```python
from build123d import *

# Parameters (mm, degrees)
ESQUISSE1_W             = 35
ESQUISSE1_H             = 35
BOSS_EXTRU_1_DEPTH      = 800
ESQUISSE2_W             = 40
ESQUISSE2_H             = 40
ESQUISSE2_W_2           = 35
ESQUISSE2_H_2           = 35
BOSS_EXTRU_2_DEPTH      = 10
ESQUISSE7_R             = 12.5
ENL_V_MAT_EXTRU_1_DEPTH = 25


with BuildPart() as part:
    # Esquisse1 → Boss.-Extru.1 (new body)
    with BuildSketch(Plane(origin=(0, 0, 0), x_dir=(0, 0, -1), z_dir=(1, 0, 0))):
        Rectangle(ESQUISSE1_W, ESQUISSE1_H)
    extrude(amount=BOSS_EXTRU_1_DEPTH)

    # Esquisse2 → Boss.-Extru.2 (add)
    # profile 1 of 2: a face of its own
    with BuildSketch(Plane.ZY):
        Rectangle(ESQUISSE2_W, ESQUISSE2_H)
        Rectangle(ESQUISSE2_W_2, ESQUISSE2_H_2, mode=Mode.SUBTRACT)
    # profile 2 of 2: a face of its own
    with BuildSketch(Plane.ZY):
        Rectangle(ESQUISSE2_W_2, ESQUISSE2_H_2)
    extrude(amount=BOSS_EXTRU_2_DEPTH)

    # Esquisse7 → Enlèv. mat.-Extru.1 (cut)
    with BuildSketch(Plane.XY.offset(17.5)):
        with Locations((770, 0)):
            Circle(ESQUISSE7_R)
    extrude(amount=-ENL_V_MAT_EXTRU_1_DEPTH, mode=Mode.SUBTRACT)


solid = part.part
```
Work out the finished part from the listing and answer in its coordinate system (mm). A direction names the side the tool comes from. Round coordinates to 2 decimals unless told otherwise and drop trailing zeros. Write each loop counter-clockwise with the first axis right and the second up, starting at its lowest first coordinate (ties: lowest second). Pieces come first, ordered by that corner, then holes. Notation, with made-up numbers: (10, 24) - (25, 24) arc R14 cw to (25, 51) - close; hole circle Ø4 at (-12.75, 65). An arc over 180 degrees is marked (long way). Return JSON: item names as keys, results as strings. Group by question number.
Q1. Find the intervals of material crossed by L1, parallel to Y at x = 770, z = 10; L2, parallel to Z at x = 595.5, y = -8, in increasing order.
Q2. The mould has two halves that part along X. Classify faces 5 (the flat face through (-10, 0, 0)), 6 (the flat face through (770, 0, -7.5)), 7 (the flat face through (394, -17.5, 0)), 8 (the flat face through (800, 0, 0)): released by +X, released by -X, zero draft, split by the parting line, or undercut.
Q3. The part is cut by section B-B on x = 770. Write down the section's boundary in (y, z), then the cut area to 3 significant figures.
Q4. The part is cut by section D-D on x = 255.5. Write down the section's boundary in (y, z).
Q5. The part is cut by section C-C on y = 0. Write down the section's boundary in (x, z).
Q6. Each of these flat-tipped pins is pushed along its axis until it touches: pin 1 Ø2 at (x, z) = (120, -12) entering from -Y; pin 2 Ø10.5 at (x, y) = (480, 7.5) entering from -Z; pin 3 Ø17.5 at (x, z) = (560.5, -4.5) entering from +Y. Where does it stop, or does it pass through?
Q7. For faces 1 (the flat face through (394, 0, -17.5)), 2 (the flat face through (394, 0, 17.5)), 3 (the flat face through (394, 17.5, 0)), 4 (the cylindrical face through (757.512, 0.55, 5.175)), determine the directions among +Z, -Z, +X, -X, +Y, -Y from which every point of the face is accessible in a straight line to the end or side of a thin tool.
Q8. The part is cut by section A-A on z = 8. Write down the section's boundary in (x, y), then the cut area to 3 significant figures.
Solved:
{
 "1": {"L1": "-17.5 to -12.5, 12.5 to 17.5", "L2": "-17.5 to 17.5"},
 "2": {"face 5": "released by -X", "face 6": "undercut", "face 7": "zero draft", "face 8": "released by +X"},
 "3": {"outline": "(-17.5, -17.5) - (17.5, -17.5) - (17.5, 17.5) - (12.5, 17.5) - (12.5, -7.5) - (-12.5, -7.5) - (-12.5, 17.5) - (-17.5, 17.5) - close", "area": "600 mm²"},
 "4": {"outline": "(-17.5, -17.5) - (17.5, -17.5) - (17.5, 17.5) - (-17.5, 17.5) - close"},
 "5": {"outline": "(-10, -20) - (0, -20) - (0, -17.5) - (800, -17.5) - (800, 17.5) - (782.5, 17.5) - (782.5, -7.5) - (757.5, -7.5) - (757.5, 17.5) - (0, 17.5) - (0, 20) - (-10, 20) - close"},
 "6": {"pin 1": "y = -17.5", "pin 2": "z = -17.5", "pin 3": "y = 17.5"},
 "7": {"face 1": "-Z, +X, +Y, -Y", "face 2": "+Z, +X, +Y, -Y", "face 3": "+Z, -Z, +X, +Y", "face 4": "+Z"},
 "8": {"outline": "(-10, -20) - (0, -20) - (0, -17.5) - (800, -17.5) - (800, 17.5) - (0, 17.5) - (0, 20) - (-10, 20) - close; hole circle Ø25 at (770, 0)", "area": "27,900 mm²"}
}
